Part model, mm, in its own coordinate system. A direction names the side the tool comes from. Coordinates: 2 decimals unless noted, no trailing zeros. Loops run counter-clockwise (first coordinate to the right, second up) from the corner with the lowest first, then second, coordinate; pieces in that order, holes last.
```python
from build123d import *

# Parameters (mm, degrees)
SKETCH_1_W          = 40
SKETCH_1_H          = 16
SKETCH_1_R          = 1.6
EXTRUDE_1_DEPTH     = 3
CHAMFER_1_SIZE      = 10
SKETCH_3_R          = 6
CUT_EXTRUDE_1_DEPTH = 10


with BuildPart() as part:
    # 草图1 → 凸台-拉伸1 (new body)
    # profile 1 of 2: a face of its own
    with BuildSketch(Plane(origin=(0, 0, 0), x_dir=(1, 0, 0), z_dir=(0, 1, 0))):
        Polygon((20, -8), (-20, -8), (-25, -8), (-25, -79), (25, -79), (25, -8), align=None)
    # profile 2 of 2: a face of its own
    with BuildSketch(Plane(origin=(0, 0, 0), x_dir=(1, 0, 0), z_dir=(0, 1, 0))):
        Rectangle(SKETCH_1_W, SKETCH_1_H)
        with Locations(Location((-11, 4, 0), (0, 0, 270))):
            Circle(SKETCH_1_R, mode=Mode.SUBTRACT)
        with Locations(Location((0, -2, 0), (0, 0, 270))):
            Circle(SKETCH_1_R, mode=Mode.SUBTRACT)
        with Locations(Location((11, 4, 0), (0, 0, 270))):
            Circle(SKETCH_1_R, mode=Mode.SUBTRACT)
    extrude(amount=EXTRUDE_1_DEPTH)

    # 倒角1
    # the kernel refuses this chamfer: 10 mm, written as the material it takes off along each edge
    with BuildSketch(Plane(origin=(-25, -25.71682988, 79), x_dir=(-0.027495876610586317, 0, -0.9996219169112968), z_dir=(0, 1, 0)), Plane(origin=(-20, -25.71682988, -8), x_dir=(0.9996219169112968, 0, -0.027495876610586317), z_dir=(0, 1, 0)), Plane(origin=(20, -25.71682988, -8), x_dir=(0.027495876610586317, 0, 0.9996219169112968), z_dir=(0, 1, 0))) as chamfer_1_piece_1:
        Polygon((CHAMFER_1_SIZE * 0.999621916911, -CHAMFER_1_SIZE * 0.0274958766106), (-CHAMFER_1_SIZE * 0.0274958766106, -CHAMFER_1_SIZE * 0.999621916911), (0, 0), align=None)
    extrude(amount=54.433659759, mode=Mode.SUBTRACT)
    with BuildSketch(Plane(origin=(-25, -25.71682988, 8), x_dir=(-0.027495876610586313, 0, 0.9996219169112968), z_dir=(0, 1, 0))) as chamfer_1_piece_2_section:
        Polygon((CHAMFER_1_SIZE * 0.999621916911, CHAMFER_1_SIZE * 0.0274958766106), (-CHAMFER_1_SIZE * 0.0274958766106, CHAMFER_1_SIZE * 0.999621916911), (0, 0), align=None)
    chamfer_1_piece_2 = extrude(amount=54.433659759, mode=Mode.PRIVATE)
    chamfer_1_piece_2 = split(chamfer_1_piece_2, bisect_by=Plane(origin=(-20, 1.5, 11.934010841), z_dir=(-1, 0, 0)), keep=Keep.TOP, mode=Mode.PRIVATE)
    add(chamfer_1_piece_2, mode=Mode.SUBTRACT)
    with BuildSketch(Plane(origin=(25, -25.71682988, 8), x_dir=(-0.9996219169112968, 0, -0.027495876610586403), z_dir=(0, 1, 0))) as chamfer_1_piece_3_section:
        Polygon((CHAMFER_1_SIZE * 0.999621916911, CHAMFER_1_SIZE * 0.0274958766106), (-CHAMFER_1_SIZE * 0.0274958766106, CHAMFER_1_SIZE * 0.999621916911), (0, 0), align=None)
    chamfer_1_piece_3 = extrude(amount=54.433659759, mode=Mode.PRIVATE)
    chamfer_1_piece_3 = split(chamfer_1_piece_3, bisect_by=Plane(origin=(20, 1.5, 11.934010841), z_dir=(1, 0, 0)), keep=Keep.TOP, mode=Mode.PRIVATE)
    add(chamfer_1_piece_3, mode=Mode.SUBTRACT)
    with BuildSketch(Plane(origin=(25, -25.71682988, 79), x_dir=(0.027495876610586317, 0, -0.9996219169112968), z_dir=(0, 1, 0))) as chamfer_1_piece_4:
        Polygon((CHAMFER_1_SIZE * 0.999621916911, CHAMFER_1_SIZE * 0.0274958766106), (-CHAMFER_1_SIZE * 0.0274958766106, CHAMFER_1_SIZE * 0.999621916911), (0, 0), align=None)
    extrude(amount=54.433659759, mode=Mode.SUBTRACT)

    # 草图3 → 切除-拉伸1 (cut)
    with BuildSketch(Plane(origin=(0, 3, 0), x_dir=(1, 0, 0), z_dir=(0, 1, 0))):
        with Locations(Location((0, -43.5, 0), (0, 0, 270))):
            Circle(SKETCH_3_R)
        with BuildLine():
            Line((-6.539230485, -52.426279442), (-10.539230485, -59.354482672))
            ThreePointArc((-10.539230485, -59.354482672), (-10.639130907, -60.113301717), (-10.173205081, -60.720508076))
            Line((-10.173205081, -60.720508076), (-9.826794919, -60.920508076))
            ThreePointArc((-9.826794919, -60.920508076), (-9.067975874, -61.020408498), (-8.460769515, -60.554482672))
            Line((-8.460769515, -60.554482672), (-4.460769515, -53.626279442))
            ThreePointArc((-4.460769515, -53.626279442), (-4.360869093, -52.867460397), (-4.826794919, -52.260254038))
            Line((-4.826794919, -52.260254038), (-5.173205081, -52.060254038))
            ThreePointArc((-5.173205081, -52.060254038), (-5.932024126, -51.960353615), (-6.539230485, -52.426279442))
        make_face()
        with BuildLine():
            Line((-0.2, -53.5), (0.2, -53.5))
            ThreePointArc((0.2, -53.5), (0.907106781, -53.792893219), (1.2, -54.5))
            Line((1.2, -54.5), (1.2, -62.5))
            ThreePointArc((1.2, -62.5), (0.907106781, -63.207106781), (0.2, -63.5))
            Line((0.2, -63.5), (-0.2, -63.5))
            ThreePointArc((-0.2, -63.5), (-0.907106781, -63.207106781), (-1.2, -62.5))
            Line((-1.2, -62.5), (-1.2, -54.5))
            ThreePointArc((-1.2, -54.5), (-0.907106781, -53.792893219), (-0.2, -53.5))
        make_face()
        with BuildLine():
            Line((-10.126279442, -47.960769515), (-17.054482672, -51.960769515))
            ThreePointArc((-17.054482672, -51.960769515), (-17.520408498, -52.567975874), (-17.420508076, -53.326794919))
            Line((-17.420508076, -53.326794919), (-17.220508076, -53.673205081))
            ThreePointArc((-17.220508076, -53.673205081), (-16.613301717, -54.139130907), (-15.854482672, -54.039230485))
            Line((-15.854482672, -54.039230485), (-8.926279442, -50.039230485))
            ThreePointArc((-8.926279442, -50.039230485), (-8.460353615, -49.432024126), (-8.560254038, -48.673205081))
            Line((-8.560254038, -48.673205081), (-8.760254038, -48.326794919))
            ThreePointArc((-8.760254038, -48.326794919), (-9.367460397, -47.860869093), (-10.126279442, -47.960769515))
        make_face()
        with BuildLine():
            Line((-11, -42.3), (-19, -42.3))
            ThreePointArc((-19, -42.3), (-19.707106781, -42.592893219), (-20, -43.3))
            Line((-20, -43.3), (-20, -43.7))
            ThreePointArc((-20, -43.7), (-19.707106781, -44.407106781), (-19, -44.7))
            Line((-19, -44.7), (-11, -44.7))
            ThreePointArc((-11, -44.7), (-10.292893219, -44.407106781), (-10, -43.7))
            Line((-10, -43.7), (-10, -43.3))
            ThreePointArc((-10, -43.3), (-10.292893219, -42.592893219), (-11, -42.3))
        make_face()
        with BuildLine():
            Line((-8.926279442, -36.960769515), (-15.854482672, -32.960769515))
            ThreePointArc((-15.854482672, -32.960769515), (-16.613301717, -32.860869093), (-17.220508076, -33.326794919))
            Line((-17.220508076, -33.326794919), (-17.420508076, -33.673205081))
            ThreePointArc((-17.420508076, -33.673205081), (-17.520408498, -34.432024126), (-17.054482672, -35.039230485))
            Line((-17.054482672, -35.039230485), (-10.126279442, -39.039230485))
            ThreePointArc((-10.126279442, -39.039230485), (-9.367460397, -39.139130907), (-8.760254038, -38.673205081))
            Line((-8.760254038, -38.673205081), (-8.560254038, -38.326794919))
            ThreePointArc((-8.560254038, -38.326794919), (-8.460353615, -37.567975874), (-8.926279442, -36.960769515))
        make_face()
        with BuildLine():
            Line((-4.460769515, -33.373720558), (-8.460769515, -26.445517328))
            ThreePointArc((-8.460769515, -26.445517328), (-9.067975874, -25.979591502), (-9.826794919, -26.079491924))
            Line((-9.826794919, -26.079491924), (-10.173205081, -26.279491924))
            ThreePointArc((-10.173205081, -26.279491924), (-10.639130907, -26.886698283), (-10.539230485, -27.645517328))
            Line((-10.539230485, -27.645517328), (-6.539230485, -34.573720558))
            ThreePointArc((-6.539230485, -34.573720558), (-5.932024126, -35.039646385), (-5.173205081, -34.939745962))
            Line((-5.173205081, -34.939745962), (-4.826794919, -34.739745962))
            ThreePointArc((-4.826794919, -34.739745962), (-4.360869093, -34.132539603), (-4.460769515, -33.373720558))
        make_face()
        with BuildLine():
            Line((1.2, -32.5), (1.2, -24.5))
            ThreePointArc((1.2, -24.5), (0.907106781, -23.792893219), (0.2, -23.5))
            Line((0.2, -23.5), (-0.2, -23.5))
            ThreePointArc((-0.2, -23.5), (-0.907106781, -23.792893219), (-1.2, -24.5))
            Line((-1.2, -24.5), (-1.2, -32.5))
            ThreePointArc((-1.2, -32.5), (-0.907106781, -33.207106781), (-0.2, -33.5))
            Line((-0.2, -33.5), (0.2, -33.5))
            ThreePointArc((0.2, -33.5), (0.907106781, -33.207106781), (1.2, -32.5))
        make_face()
        with BuildLine():
            Line((6.539230485, -34.573720558), (10.539230485, -27.645517328))
            ThreePointArc((10.539230485, -27.645517328), (10.639130907, -26.886698283), (10.173205081, -26.279491924))
            Line((10.173205081, -26.279491924), (9.826794919, -26.079491924))
            ThreePointArc((9.826794919, -26.079491924), (9.067975874, -25.979591502), (8.460769515, -26.445517328))
            Line((8.460769515, -26.445517328), (4.460769515, -33.373720558))
            ThreePointArc((4.460769515, -33.373720558), (4.360869093, -34.132539603), (4.826794919, -34.739745962))
            Line((4.826794919, -34.739745962), (5.173205081, -34.939745962))
            ThreePointArc((5.173205081, -34.939745962), (5.932024126, -35.039646385), (6.539230485, -34.573720558))
        make_face()
        with BuildLine():
            Line((10.126279442, -39.039230485), (17.054482672, -35.039230485))
            ThreePointArc((17.054482672, -35.039230485), (17.520408498, -34.432024126), (17.420508076, -33.673205081))
            Line((17.420508076, -33.673205081), (17.220508076, -33.326794919))
            ThreePointArc((17.220508076, -33.326794919), (16.613301717, -32.860869093), (15.854482672, -32.960769515))
            Line((15.854482672, -32.960769515), (8.926279442, -36.960769515))
            ThreePointArc((8.926279442, -36.960769515), (8.460353615, -37.567975874), (8.560254038, -38.326794919))
            Line((8.560254038, -38.326794919), (8.760254038, -38.673205081))
            ThreePointArc((8.760254038, -38.673205081), (9.367460397, -39.139130907), (10.126279442, -39.039230485))
        make_face()
        with BuildLine():
            Line((11, -44.7), (19, -44.7))
            ThreePointArc((19, -44.7), (19.707106781, -44.407106781), (20, -43.7))
            Line((20, -43.7), (20, -43.3))
            ThreePointArc((20, -43.3), (19.707106781, -42.592893219), (19, -42.3))
            Line((19, -42.3), (11, -42.3))
            ThreePointArc((11, -42.3), (10.292893219, -42.592893219), (10, -43.3))
            Line((10, -43.3), (10, -43.7))
            ThreePointArc((10, -43.7), (10.292893219, -44.407106781), (11, -44.7))
        make_face()
        with BuildLine():
            Line((8.926279442, -50.039230485), (15.854482672, -54.039230485))
            ThreePointArc((15.854482672, -54.039230485), (16.613301717, -54.139130907), (17.220508076, -53.673205081))
            Line((17.220508076, -53.673205081), (17.420508076, -53.326794919))
            ThreePointArc((17.420508076, -53.326794919), (17.520408498, -52.567975874), (17.054482672, -51.960769515))
            Line((17.054482672, -51.960769515), (10.126279442, -47.960769515))
            ThreePointArc((10.126279442, -47.960769515), (9.367460397, -47.860869093), (8.760254038, -48.326794919))
            Line((8.760254038, -48.326794919), (8.560254038, -48.673205081))
            ThreePointArc((8.560254038, -48.673205081), (8.460353615, -49.432024126), (8.926279442, -50.039230485))
        make_face()
        with BuildLine():
            Line((4.460769515, -53.626279442), (8.460769515, -60.554482672))
            ThreePointArc((8.460769515, -60.554482672), (9.067975874, -61.020408498), (9.826794919, -60.920508076))
            Line((9.826794919, -60.920508076), (10.173205081, -60.720508076))
            ThreePointArc((10.173205081, -60.720508076), (10.639130907, -60.113301717), (10.539230485, -59.354482672))
            Line((10.539230485, -59.354482672), (6.539230485, -52.426279442))
            ThreePointArc((6.539230485, -52.426279442), (5.932024126, -51.960353615), (5.173205081, -52.060254038))
            Line((5.173205081, -52.060254038), (4.826794919, -52.260254038))
            ThreePointArc((4.826794919, -52.260254038), (4.360869093, -52.867460397), (4.460769515, -53.626279442))
        make_face()
    extrude(amount=-CUT_EXTRUDE_1_DEPTH, mode=Mode.SUBTRACT)


solid = part.part
```
Q1. Tool access for faces 1 (the flat face through (20, 1, 8)), 2 (the flat face through (6.43, 1.52, 57.04)), 3 (the flat face through (25, 1, 44)): list every direction of +Z, -Z, +X, -X, +Y, -Y with a clear straight run to the whole face (end or side of a thin tool).
Q2. Mould opens along Z. For faces 4 (the flat face through (0, 0, 35)), 5 (the flat face through (20, 1, 74)), 6 (the flat face through (-23, 1, 16)), 7 (the flat face through (-12.44, 1.52, 52.07)) say: released by +Z, released by -Z, zero draft, split by the parting line, or undercut.
Q3. Saw through at A-A (x = -13.5). List the corners of the cut face in (y, z), plus the area to 3 significant figures.
Q4. Probe line 1 (X direction, y = 0.9, z = 43.5); line 2 (Z direction, x = -15, y = 0.95); line 3 (X direction, y = 1.3, z = 36). List the from-to ranges inside material, lowest first.
Q5. Saw through at B-B (y = 2.15). Count the separate pieces of the cut face and the enclosed holes in it, plus the area to 3 significant figures.
Q6. Drop flat-ended pins along their axis: P1, Ø1.5, axis at x = 16.5, y = 1.5, coming from the +Z side; P2, Ø1, axis at x = 14, y = 2, coming from the -Z side; P3, Ø1.5, axis at y = 1, z = 5.5, coming from the -X side. Give the stop position or say it passes through.
Checked values:
1. face 1: -Z, +X, +Y, -Y
1. face 2: +Y, -Y
1. face 3: +Z, -Z, +X, +Y, -Y
2. face 4: zero draft
2. face 5: released by +Z
2. face 6: released by -Z
2. face 7: undercut
3. outline: (0, -4.5) - (3, -4.5) - (3, 34.32) - (0, 34.32) - close; (0, 37.09) - (3, 37.09) - (3, 42.3) - (0, 42.3) - close; (0, 44.7) - (3, 44.7) - (3, 49.91) - (0, 49.91) - close; (0, 52.68) - (3, 52.68) - (3, 79) - (0, 79) - close
3. area: 227 mm2
4. line 1: x = -25 to -20, -10 to -6, 6 to 10, 20 to 25
4. line 2: z = -3 to 33.45, 36.23 to 42.3, 44.7 to 50.77, 53.55 to 79
4. line 3: x = -25 to -15.39, -10.59 to 10.59, 15.39 to 25
5. separate pieces: 1
5. enclosed holes: 16
5. area: 3,500 mm2
6. P1: stops at z = 78.25
6. P2: stops at z = -4.5
6. P3: stops at x = -20
